from build123d import *

# Parameters (mm, degrees)
F0_R     = 10
F0_R_2   = 4.25
F1_DEPTH = 10.2
F3_R     = 10
F3_R_2   = 3
F4_DEPTH = 1
F7_DEPTH = 15


with BuildPart() as f1:
    # F0 (on Top) → F1 (new body)
    with BuildSketch(Plane.XY):
        Circle(F0_R)
        Circle(F0_R_2, mode=Mode.SUBTRACT)
    extrude(amount=F1_DEPTH)

    # F3 (on offset) → F4 (join)
    with BuildSketch(Plane.XY.offset(10.2)):
        Circle(F3_R)
        Circle(F3_R_2, mode=Mode.SUBTRACT)
    extrude(amount=F4_DEPTH)

    # F6 (on offset) → F7 (cut)
    with BuildSketch(Plane.XY.offset(11.2)):
        with BuildLine():
            ThreePointArc((0, -5.5), (-1.5, -7), (0, -8.5))
            Line((0, -8.5), (0, -5.5))
        make_face()
        with BuildLine():
            ThreePointArc((0, 8.5), (-1.5, 7), (0, 5.5))
            Line((0, 5.5), (0, 8.5))
        make_face()
        with BuildLine():
            Line((0, 8.5), (0, 5.5))
            ThreePointArc((0, 5.5), (1.06066, 5.93934), (1.5, 7))
            ThreePointArc((1.5, 7), (1.06066, 8.06066), (0, 8.5))
        make_face()
        with BuildLine():
            Line((0, -5.5), (0, -8.5))
            ThreePointArc((0, -8.5), (1.06066, -8.06066), (1.5, -7))
            ThreePointArc((1.5, -7), (1.06066, -5.93934), (0, -5.5))
        make_face()
    extrude(amount=-F7_DEPTH, mode=Mode.SUBTRACT)


solid = f1.part
Verification items for the finished model (mm, model axes). A direction names the side the tool comes from. Coordinates: 2 decimals unless noted, no trailing zeros. Write each loop counter-clockwise with the first axis right and the second up, starting at its lowest first coordinate (ties: lowest second). Pieces come first, ordered by that corner, then holes. Notation, with made-up numbers: (-22.75, -28.5) -> (-15.75, -28.5) arc R11 cw to (-15.75, -23.5) -> close; hole circle Ø8 at (47.25, 50). An arc over 180 degrees is marked (long way). One line per item, written item: value. Start each with the question number.
Q1. Cross-section at B-B on z = 8.5. Enter the section's corners in (x, y).
Q2. Cross-section at A-A on y = 0. Enter the section's corners in (x, z).
Q3. Go/stop test with flat-tipped pins: P1, Ø5, axis at y = -6, z = 7, coming from the -X side; P2, Ø5, axis at x = 7, z = 1.5, coming from the +Y side; P3, Ø4, axis at x = 3.5, z = 10, coming from the +Y side. Record where each tip stops, or that it passes through.
Q4. Cross-section at D-D on y = 7.75. Enter the section's corners in (x, z), and give its area (3 significant figures).
Q5. Thickness scan on L1, parallel to X at y = 7.5, z = 8; L2, parallel to X at y = -3.5, z = 3; L3, parallel to Y at x = -2.25, z = 6. Record the ranges inside material, lowest first. Write a range as from..to.
Q6. Mould release check, pull along X, two halves, no side actions. Record for faces 3 (the cylindrical face through (2.285, 3.584, 5.029)), 4 (the cylindrical face through (-2.17, -9.76, 5.52)), 5 (the flat face through (4, -2, 0)): pulls with the +X half, pulls with the -X half, needs draft (parallel to the pull), parting line crosses it, or undercut.
Q7. Access from +Z, -Z, +X, -X, +Y, -Y to the whole of each face (thin tool, end or side, straight path). Record for faces 1 (the cylindrical face through (-3, 0, 11)), 2 (the flat face through (1, 3, 10.2)).
Q8. Cross-section at C-C on x = -2.75. Enter the section's corners in (y, z), and give its area (3 significant figures).
Checked values:
1. outline: circle Ø20 at (0, 0); hole circle Ø8.5 at (0, 0); hole (0, -5.5) arc R1.5 ccw (long way) to (1.5, -7) arc R1.5 ccw to start; hole (0, 8.5) arc R1.5 ccw (long way) to (1.5, 7) arc R1.5 ccw to start
2. outline: (-10, 0) -> (-4.25, 0) -> (-4.25, 10.2) -> (-3, 10.2) -> (-3, 11.2) -> (-10, 11.2) -> close; (3, 10.2) -> (4.25, 10.2) -> (4.25, 0) -> (10, 0) -> (10, 11.2) -> (3, 11.2) -> close
3. P1: stops at x = -9.37
3. P2: stops at y = 8.93
3. P3: stops at y = 9.89
4. outline: (-6.32, 0) -> (-1.3, 0) -> (-1.3, 11.2) -> (-6.32, 11.2) -> close; (1.3, 0) -> (6.32, 0) -> (6.32, 11.2) -> (1.3, 11.2) -> close
4. area: 112 mm²
5. L1: x = -6.61..-1.41, 1.41..6.61
5. L2: x = -9.37..-2.41, 2.41..9.37
5. L3: y = -9.74..-3.61, 3.61..9.74
6. face 3: undercut
6. face 4: parting line crosses it
6. face 5: needs draft
7. face 1: +Z, -Z
7. face 2: -Z
8. outline: (-9.61, 0) -> (-3.24, 0) -> (-3.24, 10.2) -> (-1.2, 10.2) -> (-1.2, 11.2) -> (-9.61, 11.2) -> close; (1.2, 10.2) -> (3.24, 10.2) -> (3.24, 0) -> (9.61, 0) -> (9.61, 11.2) -> (1.2, 11.2) -> close
8. area: 147 mm²
